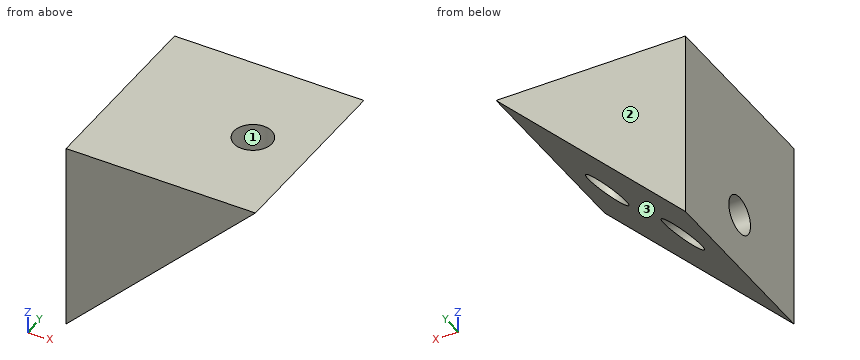
from build123d import *

# Parameters (mm, degrees)
BOSS_EXTRUDE1_DEPTH = 20
SKETCH2_R           = 2
CUT_EXTRUDE1_DEPTH  = 35.641016151


with BuildPart() as part:
    # Sketch1 → Boss-Extrude1 (new body)
    with BuildSketch(Plane(origin=(0, 0, 0), x_dir=(1, 0, 0), z_dir=(0, 1, 0))):
        Polygon((0, 20), (0, 0), (20, 0), align=None)
    extrude(amount=BOSS_EXTRUDE1_DEPTH)

    # Sketch2 → Cut-Extrude1 (cut, through all)
    with BuildSketch(Plane.XY):
        with Locations((14, 10)):
            Circle(SKETCH2_R)
    cut_extrude1 = extrude(amount=-CUT_EXTRUDE1_DEPTH, mode=Mode.SUBTRACT)

    # Mirror1: Cut-Extrude1 across plane
    add(cut_extrude1.mirror(Plane(origin=(0, 0, 0), x_dir=(-0.7071067811865475, 0, 0.7071067811865476), z_dir=(0.7071067811865478, 0, 0.7071067811865474))), mode=Mode.SUBTRACT)


solid = part.part
CAD build for the part. Positions are in the model's coordinates, mm. Face numbers are marked on the shaded views. Give positions to 0.01 mm unless a question says otherwise; leave off trailing zeros. Write each loop counter-clockwise with the first axis right and the second up, starting at its lowest first coordinate (ties: lowest second). Pieces come first, ordered by that corner, then holes. Notation, with made-up numbers: (23, 25.25) - (71, 25.25) arc R19 ccw to (71, 35.25) - close; hole circle Ø8 at (24, 27). An arc over 180 degrees is marked (long way). Answer as CSV lines item,"result".
Q1. Band-saw the part on A-A (x = 14). Give the cut face in (y, z).
Result set:
outline,"(0, -6) - (8, -6) - (8, 0) - (0, 0) - close; (12, -6) - (20, -6) - (20, 0) - (12, 0) - close"
Q2. Pull direction X, two halves, no side cores. Call the marked faces 1, 2 and 3: released by +X, released by -X, zero draft, split by the parting line, or undercut.
Result set:
face 1,"undercut"
face 2,"zero draft"
face 3,"released by +X"
Q3. Flat gauge pins, fed straight in: pin 1 Ø8 at (y, z) = (9.5, -16) entering from +X; pin 2 Ø4.5 at (y, z) = (10, -14) entering from +X; pin 3 Ø4.5 at (x, y) = (14, 10) entering from -Z. Where does each tip first touch, or does it go through?
Result set:
pin 1,"x = 8"
pin 2,"x = 8.25"
pin 3,"z = -8.25"
Q4. Band-saw the part on C-C (z = -14). Give the cut face in (x, y).
Result set:
outline,"(0, 0) - (6, 0) - (6, 8) - (0, 8) - close; (0, 12) - (6, 12) - (6, 20) - (0, 20) - close"
Q5. Band-saw the part on D-D (z = -2.75). Give the cut face in (x, y).
Result set:
outline,"(0, 0) - (17.25, 0) - (17.25, 20) - (0, 20) - close; hole circle Ø4 at (14, 10)"
Q6. Band-saw the part on B-B (y = 10). Give the cut face in (x, z), and give its area (3 significant figures).
Result set:
outline,"(0, -20) - (4, -16) - (0, -16) - close; (0, -12) - (8, -12) - (12, -8) - (12, 0) - (0, 0) - close; (16, -4) - (20, 0) - (16, 0) - close"
area,"152 mm²"
Q7. Drill centre lines: line 1 (Y direction, x = 1.75, z = -14); line 2 (X direction, y = 10, z = -2.5); line 3 (X direction, y = 18, z = -8). Where is each one in solid material? Low to high. Write a range as from..to.
Result set:
line 1,"0..8, 12..20"
line 2,"0..12, 16..17.5"
line 3,"0..12"
